from build123d import *

# Parameters (mm, degrees)
F0_R     = 5.08
F1_DEPTH = 12.7
F3_DEPTH = 25.4
F4_R     = 5.08
F5_DEPTH = 3.175
F6_R     = 5.08
F7_DEPTH = 3.175
F8_R     = 3.175
F9_DEPTH = 3.175


with BuildPart() as f1:
    # F0 (on Top) → F1 (new body)
    with BuildSketch(Plane.XY):
        Circle(F0_R)
    extrude(amount=F1_DEPTH)

    # F2 (on face) → F3 (cut)
    with BuildSketch(Plane.XY.offset(12.7)):
        with BuildLine():
            Line((1.5875, -2.749631), (1.5875, 2.749631))
            ThreePointArc((1.5875, 2.749631), (-3.175, 0), (1.5875, -2.749631))
        make_face()
    extrude(amount=-F3_DEPTH, mode=Mode.SUBTRACT)

    # F4 (on face) → F5 (join)
    with BuildSketch(Plane.XY.offset(12.7)):
        Circle(F4_R)
    extrude(amount=F5_DEPTH)

    # F6 (on face) → F7 (join)
    with BuildSketch(Plane(origin=(0, 0, 0), x_dir=(1, 0, 0), z_dir=(0, 0, -1))):
        Circle(F6_R)
    extrude(amount=F7_DEPTH)

    # F8 (on face) → F9 (cut)
    with BuildSketch(Plane(origin=(0, 0, -3.175), x_dir=(1, 0, 0), z_dir=(0, 0, -1))):
        Circle(F8_R)
    extrude(amount=-F9_DEPTH, mode=Mode.SUBTRACT)


solid = f1.part
Verification items for the finished model (mm, model axes). A direction names the side the tool comes from. Round coordinates to 2 decimals unless told otherwise and drop trailing zeros. Loops run counter-clockwise (first coordinate to the right, second up) from the corner with the lowest first, then second, coordinate; pieces in that order, holes last. Notation, with made-up numbers: (30, 24.5) - (62, 24.5) arc R17 ccw to (62, 50.5) - close; hole circle Ø1 at (45.25, 28). An arc over 180 degrees is marked (long way). Answer in a Markdown table with one row per item. Add a question column.
Q1. Gauge pin test, flat ends, axial feed: pin 1 (3 mm diameter, centred on y = 3.5, z = 12, fed in from +X); pin 2 (0.8 mm diameter, centred on x = 2.5, y = 0.5, fed in from -Z); pin 3 (2 mm diameter, centred on y = 1.5, z = 3, fed in from +X). Record the tip position at first contact, or that the pin passes through.
Q2. Section check C-C on y = 0. Enter the section's corners in (x, z) (1 decimal).
Q3. Release check for a two-part mould opening along Y. For faces 1 (the face through (-0.661, -5.037, 6.483)), 2 (the face through (0, 0, 12.7)), 3 (the face through (0, 0, 15.875)), 4 (the face through (2, 0, 0)) record: pulls with the +Y half, pulls with the -Y half, needs draft (parallel to the pull), parting line crosses it, or undercut.
Q4. Tool access check on faces 5 (the face through (3.3, 1.1, -3.175)), 6 (the face through (1.588, 0, 6)). Record the directions out of +Z, -Z, +X, -X, +Y, -Y that give a thin tool (end or side, any length) a straight path to the whole face; none if there is none.
Q5. Section check D-D on z = 13. Enter the section's corners in (x, y).
Q6. Section check A-A on x = 0. Enter the section's corners in (y, z) (3 decimals), plus the area to 3 significant figures.
Q7. Material ranges on line 1 (Y direction, x = 0, z = -1.65) (3 decimals); line 2 (Z direction, x = -2.5, y = 1) (3 decimals), recorded low to high.
Found:
| question | item | result |
|---|---|---|
| 1 | pin 1 | stops at x = 4.67 |
| 1 | pin 2 | stops at z = 0 |
| 1 | pin 3 | stops at x = 5.06 |
| 2 | outline | (-5.1, -3.2) - (-3.2, -3.2) - (-3.2, 12.7) - (1.6, 12.7) - (1.6, 0) - (3.2, 0) - (3.2, -3.2) - (5.1, -3.2) - (5.1, 15.9) - (-5.1, 15.9) - close |
| 3 | face 1 | parting line crosses it |
| 3 | face 2 | undercut |
| 3 | face 3 | needs draft |
| 3 | face 4 | undercut |
| 4 | face 5 | -Z, +X, -X, +Y, -Y |
| 4 | face 6 | -Z |
| 5 | outline | circle Ø10.16 at (0, 0) |
| 6 | outline | (-5.08, -3.175) - (-3.175, -3.175) - (-3.175, 12.7) - (3.175, 12.7) - (3.175, -3.175) - (5.08, -3.175) - (5.08, 15.875) - (-5.08, 15.875) - close |
| 6 | area | 92.7 mm² |
| 7 | line 1 | y = -5.08 to -3.175, 3.175 to 5.08 |
| 7 | line 2 | z = 12.7 to 15.875 |
